For this review, take the finished solid that the model builds, in its own axes (mm). Face numbers are marked on the shaded views. A direction names the side the tool comes from. Give positions to 0.01 mm unless a question says otherwise; leave off trailing zeros. Write each loop counter-clockwise with the first axis right and the second up, starting at its lowest first coordinate (ties: lowest second). Pieces come first, ordered by that corner, then holes.
Q1. We need section D-D (x = -6.5). Write out the cut boundary in (y, z).
Q2. Mouldability with a two-part tool opening along Z and no side actions: class the marked faces 6, 7 and 8 as released by +Z, released by -Z, zero draft, split by the parting line, or undercut.
Q3. For line 1 (Y direction, x = 29, z = -0.5); line 2 (Z direction, x = -32, y = 22.5); line 3 (Y direction, x = 12.5, z = 0), list the stretches that pass through material, from the lowest coordinate up.
Q4. We need section B-B (y = 42.5). Write out the cut boundary in (x, z).
Q5. Insertion check: P1, Ø8, axis at x = 33.5, y = 43, coming from the +Z side; P2, Ø1.5, axis at x = 28.5, y = 48, coming from the +Z side; P3, Ø1, axis at x = 32.5, z = -16, coming from the +Y side; P4, Ø9.5, axis at x = -21, y = 30, coming from the +Z side. Each pin has a flat end and moves straight along its axis. Give the tip position at first contact, or say it passes through.
Q6. We need section A-A (x = -21). Write out the cut boundary in (y, z).
Q7. We need section C-C (z = 2.5). Write out the cut boundary in (x, y).
Q8. Machinability: for the marked faces 1, 2, 3, 4 and 5, which of the approach directions +Z, -Z, +X, -X, +Y, -Y give a long, thin tool a straight path to every point of the face, cutting with its end or side? Answer none if there is none.
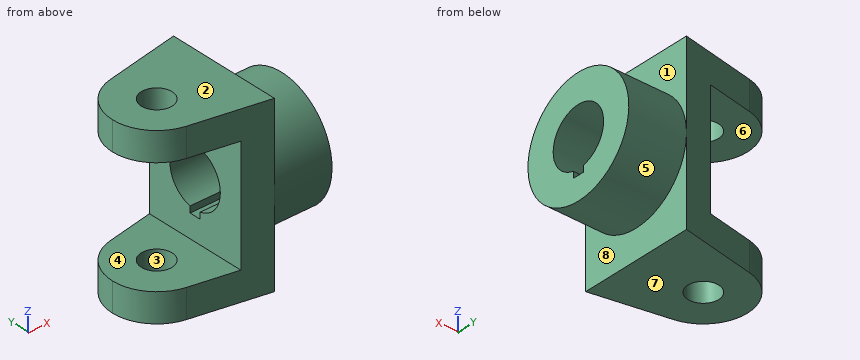
```python
from build123d import *

# Parameters (mm, degrees)
SKETCH1_W           = 88
SKETCH1_H           = 90
BOSS_EXTRUDE1_DEPTH = 60
SKETCH2_W           = 43
SKETCH2_H           = 60
SKETCH2_W_2         = 30
SKETCH2_H_2         = 90
CUT_EXTRUDE1_DEPTH  = 60
SKETCH3_R           = 8
CUT_EXTRUDE2_DEPTH  = 125
CUT_EXTRUDE3_DEPTH  = 30
SKETCH4_4_R         = 30
BOSS_EXTRUDE2_DEPTH = 30


with BuildPart() as part:
    # Sketch1 → Boss-Extrude1 (new body)
    with BuildSketch(Plane(origin=(0, 0, 0), x_dir=(1, 0, 0), z_dir=(0, 1, 0))):
        Rectangle(SKETCH1_W, SKETCH1_H)
    extrude(amount=BOSS_EXTRUDE1_DEPTH)

    # Sketch2 → Cut-Extrude1 (cut)
    with BuildSketch(Plane(origin=(0, 60, 0), x_dir=(1, 0, 0), z_dir=(0, 1, 0))):
        with Locations((-22.5, 0)):
            Rectangle(SKETCH2_W, SKETCH2_H)
        with Locations((29, 0)):
            Rectangle(SKETCH2_W_2, SKETCH2_H_2)
    extrude(amount=-CUT_EXTRUDE1_DEPTH, mode=Mode.SUBTRACT)

    # Sketch3 → Cut-Extrude2 (cut)
    with BuildSketch(Plane.XY.offset(45)):
        with BuildLine():
            ThreePointArc((-25.259048664, 7.397776559), (-38.705339862, 15.31936853), (-44, 30))
            Line((-44, 30), (-44, 0))
            Line((-44, 0), (14, 0))
            Line((14, 0), (-25.259048664, 7.397776559))
        make_face()
        with BuildLine():
            ThreePointArc((-44, 30), (-38.705339862, 44.68063147), (-25.259048664, 52.602223441))
            Line((-25.259048664, 52.602223441), (14, 60))
            Line((14, 60), (-44, 60))
            Line((-44, 60), (-44, 30))
        make_face()
        with Locations((-21, 30)):
            Circle(SKETCH3_R)
    extrude(amount=-CUT_EXTRUDE2_DEPTH, mode=Mode.SUBTRACT)

    # Sketch4 → Cut-Extrude3 (cut)
    with BuildSketch(Plane(origin=(14, 0, 0), x_dir=(0, 0, -1), z_dir=(1, 0, 0))):
        with BuildLine():
            Line((14.696938457, 33), (18, 33))
            Line((18, 33), (18, 27))
            Line((18, 27), (14.696938457, 27))
            ThreePointArc((14.696938457, 27), (-15, 30), (14.696938457, 33))
        make_face()
    extrude(amount=-CUT_EXTRUDE3_DEPTH, mode=Mode.SUBTRACT)

    # Sketch4_4 → Boss-Extrude2 (add)
    with BuildSketch(Plane(origin=(14, 0, 0), x_dir=(0, 0, -1), z_dir=(1, 0, 0))):
        with Locations((0, 30)):
            Circle(SKETCH4_4_R)
        with BuildLine():
            Line((14.696938457, 33), (18, 33))
            Line((18, 33), (18, 27))
            Line((18, 27), (14.696938457, 27))
            ThreePointArc((14.696938457, 27), (-15, 30), (14.696938457, 33))
        make_face(mode=Mode.SUBTRACT)
    extrude(amount=BOSS_EXTRUDE2_DEPTH)


solid = part.part
```
Computed:
1. outline: (3.86, -45) - (56.14, -45) - (56.14, -30) - (3.86, -30) - close; (3.86, 30) - (56.14, 30) - (56.14, 45) - (3.86, 45) - close
2. face 6: undercut
2. face 7: released by -Z
2. face 8: zero draft
3. line 1: y = 0 to 15.01, 44.99 to 60
3. line 2: z = -45 to -30, 30 to 45
3. line 3: y = 0.28 to 15, 45 to 59.72
4. outline: (-40.31, -45) - (14, -45) - (14, -27.27) - (44, -27.27) - (44, -8.29) - (-1, -8.29) - (-1, -30) - (-40.31, -30) - close; (-40.31, 30) - (-1, 30) - (-1, 8.29) - (44, 8.29) - (44, 27.27) - (14, 27.27) - (14, 45) - (-40.31, 45) - close
5. P1: stops at z = 28.62
5. P2: stops at z = 24.54
5. P3: stops at y = 55.69
5. P4: passes through
6. outline: (6.6, -45) - (22, -45) - (22, -30) - (6.6, -30) - close; (6.6, 30) - (22, 30) - (22, 45) - (6.6, 45) - close; (38, -45) - (53.4, -45) - (53.4, -30) - (38, -30) - close; (38, 30) - (53.4, 30) - (53.4, 45) - (38, 45) - close
7. outline: (-1, 2.83) - (14, 0) - (14, 0.1) - (44, 0.1) - (44, 15.21) - (-1, 15.21) - close; (-1, 44.79) - (44, 44.79) - (44, 59.9) - (14, 59.9) - (14, 60) - (-1, 57.17) - close
8. face 1: +Z, +X
8. face 2: +Z, +X, -X, +Y, -Y
8. face 3: +Z, -Z
8. face 4: -X, +Y, -Y
8. face 5: +X
